```python
from build123d import *

# Parameters (mm, degrees)
SKETCH_1_R          = 5
SKETCH_1_R_2        = 1.5
EXTRUDE_1_DEPTH     = 1
SKETCH_2_R          = 4
EXTRUDE_2_DEPTH     = 2
SKETCH_3_R          = 1.5
CUT_EXTRUDE_1_DEPTH = 8.681145748


with BuildPart() as part:
    # 스케치1 → 돌출1 (new body)
    with BuildSketch(Plane.XY):
        Circle(SKETCH_1_R)
        Circle(SKETCH_1_R_2, mode=Mode.SUBTRACT)
    extrude(amount=EXTRUDE_1_DEPTH)

    # 스케치2 → 돌출2 (add)
    with BuildSketch(Plane.XY.offset(1)):
        Circle(SKETCH_2_R)
    extrude(amount=EXTRUDE_2_DEPTH)

    # 스케치3 → 컷-돌출1 (cut, through all)
    with BuildSketch(Plane.XY.offset(3)):
        Circle(SKETCH_3_R)
    extrude(amount=-CUT_EXTRUDE_1_DEPTH, mode=Mode.SUBTRACT)


solid = part.part
```
CAD build for the part. Positions are in the model's coordinates, mm. Round coordinates to 2 decimals unless told otherwise and drop trailing zeros. Order: outer loops, then holes, each group sorted by start corner. A loop starts at its lowest first (then second) coordinate and runs counter-clockwise, first axis right, second up. Notation, with made-up numbers: (88, 79.5) -> (106, 79.5) arc R17 ccw to (106, 103.5) -> close; hole circle Ø4 at (35, 53.25). An arc over 180 degrees is marked (long way). Write item = value, one per line.
(1) Cut at D-D (y = 3.75). Write the cut outline in (x, z), plus the area to 3 significant figures.
Answers follow:
outline = (-3.31, 0) -> (3.31, 0) -> (3.31, 1) -> (1.39, 1) -> (1.39, 3) -> (-1.39, 3) -> (-1.39, 1) -> (-3.31, 1) -> close
area = 12.2 mm²
(2) Cut at C-C (z = 1.3). Write the cut outline in (x, y).
Answers follow:
outline = circle Ø8 at (0, 0); hole circle Ø3 at (0, 0)
(3) Cut at A-A (x = 0). Write the cut outline in (y, z).
Answers follow:
outline = (-5, 0) -> (-1.5, 0) -> (-1.5, 3) -> (-4, 3) -> (-4, 1) -> (-5, 1) -> close; (1.5, 0) -> (5, 0) -> (5, 1) -> (4, 1) -> (4, 3) -> (1.5, 3) -> close
(4) Pull direction Y, two halves, no side cores. Call faces 1 (the cylindrical face through (-0.867, -3.905, 1.986)), 2 (the cylindrical face through (-1.5, 0.07, 1.52)), 3 (the flat face through (-1.2, 1.2, 0)): +Y half, -Y half, draft (parallel to the pull), parting line (faces both ways), or undercut.
Answers follow:
face_1 = parting line
face_2 = undercut
face_3 = draft
(5) Drill centre lines: L1, parallel to Y at x = -0.75, z = 2.2; L2, parallel to X at y = -0.5, z = 2.85; L3, parallel to Y at x = 3, z = 0.45. Where is each one in solid material? Low to high.
Answers follow:
L1 = -3.93 to -1.3, 1.3 to 3.93
L2 = -3.97 to -1.41, 1.41 to 3.97
L3 = -4 to 4
(6) Flat gauge pins, fed straight in: P1, Ø1, axis at x = -2.5, z = 1, coming from the +Y side; P2, Ø1.5, axis at y = -2.5, z = 2, coming from the +X side; P3, Ø1, axis at x = 3.5, z = 2.5, coming from the -Y side. Where does each tip first touch, or does it go through?
Answers follow:
P1 = 4.58
P2 = 3.6
P3 = -2.65
